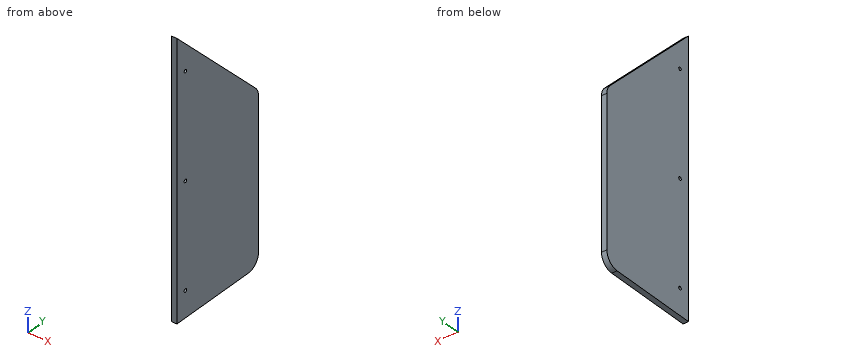
from build123d import *

# Parameters (mm, degrees)
SKETCH1_R           = 1.5
BOSS_EXTRUDE1_DEPTH = 5
FILLET1_R           = 12


with BuildPart() as part:
    # Sketch1 → Boss-Extrude1 (new body)
    with BuildSketch(Plane(origin=(0, 0, 0), x_dir=(0, 0, -1), z_dir=(1, 0, 0))):
        Polygon((0, 0), (0, 96), (-154, 96), (-250, 0), align=None)
        with Locations((-120, 10)):
            Circle(SKETCH1_R, mode=Mode.SUBTRACT)
        with Locations((-24, 10)):
            Circle(SKETCH1_R, mode=Mode.SUBTRACT)
        with Locations((-216, 10)):
            Circle(SKETCH1_R, mode=Mode.SUBTRACT)
    extrude(amount=BOSS_EXTRUDE1_DEPTH)

    # Fillet1
    fillet1_edges = [part.edges().sort_by_distance(p)[0] for p in [
        (2.5, 96, 154),
        (2.5, 96, 0),
    ]]
    fillet(fillet1_edges, radius=FILLET1_R)


solid = part.part
Read the model definition and answer for the solid it produces. Units are mm, in the model's axes. Coordinates: 2 decimals unless noted, no trailing zeros. Loops run counter-clockwise (first coordinate to the right, second up) from the corner with the lowest first, then second, coordinate; pieces in that order, holes last. Notation, with made-up numbers: (70, 32.5) -> (95, 32.5) arc R30 cw to (95, 64.5) -> close; hole circle Ø2 at (75.5, 80.5). An arc over 180 degrees is marked (long way). Answer in a Markdown table with one row per item.
Item 1: Straight lines are drawn through the part: line 1 along Z through (x, y) = (1.8, 9.5); line 2 along Y through (x, z) = (1.6, 120); line 3 along Z through (x, y) = (4.05, 9). For each, find the intervals that lie inside material, in ascending order. Write a range as [from, to].
Returned:
| item | result |
|---|---|
| line 1 | z = [0, 22.59], [25.41, 118.59], [121.41, 214.59], [217.41, 240.5] |
| line 2 | y = [0, 8.5], [11.5, 96] |
| line 3 | z = [0, 22.88], [25.12, 118.88], [121.12, 214.88], [217.12, 241] |
Item 2: A cutting plane is placed at A-A on x = 4.1. Determine the outline of the cut face in (y, z), plus the area to 3 significant figures.
Returned:
| item | result |
|---|---|
| outline | (0, 0) -> (84, 0) arc R12 ccw to (96, 12) -> (96, 149.03) arc R12 ccw to (92.49, 157.51) -> (0, 250) -> close; hole circle Ø3 at (10, 24); hole circle Ø3 at (10, 120); hole circle Ø3 at (10, 216) |
| area | 19,300 mm^2 |
Item 3: A cutting plane is placed at C-C on z = 208.5. Determine the outline of the cut face in (x, y), plus the area to 4 significant figures.
Returned:
| item | result |
|---|---|
| outline | (0, 0) -> (5, 0) -> (5, 41.5) -> (0, 41.5) -> close |
| area | 207.5 mm^2 |
Item 4: A cutting plane is placed at B-B on y = 28. Determine the outline of the cut face in (x, z).
Returned:
| item | result |
|---|---|
| outline | (0, 0) -> (5, 0) -> (5, 222) -> (0, 222) -> close |
